```python
from build123d import *

# Parameters (mm, degrees)
F0_R     = 23.199373
F1_DEPTH = 12.7
F2_R     = 23.199373
F3_DEPTH = 12.7
F4_R     = 5.08


with BuildPart() as f1:
    # F0 (on Front) → F1 (new body)
    with BuildSketch(Plane.XZ):
        with Locations((-16.925193, -16.925193)):
            Circle(F0_R)
    extrude(amount=F1_DEPTH)

    # F2 (on face) → F3 (join)
    with BuildSketch(Plane(origin=(0, 0, 0), x_dir=(-1, 0, 0), z_dir=(0, 1, 0))):
        with Locations((16.925193, -16.925193)):
            Circle(F2_R)
    extrude(amount=F3_DEPTH)

    # F4
    f4_edges = [f1.edges().sort_by_distance(p)[0] for p in [
        (6.274179, 12.7, -16.925193),
        (-16.925193, 0, 6.274179),
        (-16.925193, 0, -40.124566),
        (6.274179, -6.35, -16.925193),
        (-40.124566, -12.7, -16.925193),
        (-40.124566, 6.35, -16.925193),
    ]]
    fillet(f4_edges, radius=F4_R)


solid = f1.part
```
Geometry: final body of the model. Coordinates: model frame, mm. Round coordinates to 2 decimals unless told otherwise and drop trailing zeros. Write each loop counter-clockwise with the first axis right and the second up, starting at its lowest first coordinate (ties: lowest second). Pieces come first, ordered by that corner, then holes. Notation, with made-up numbers: (-33.75, 49.5) -> (-13.75, 49.5) arc R24 ccw to (-13.75, 78.5) -> close; hole circle Ø9 at (81.25, 17). An arc over 180 degrees is marked (long way). Use CSV: the item, a comma, the result in double quotes. Start each with the question number.
Q1. Line query: L1, parallel to X at y = 10.5, z = -32; L2, parallel to Z at x = -28.5, y = 5.25; L3, parallel to Z at x = -14, y = 2. Output: solid intervals per line, ascending.
Q2. Section A-A (y = 10.25). Return loops of the section in (x, z), plus the area to 3 significant figures.
Q3. First-contact query: pin 1 Ø12 at (x, y) = (-20.5, 2) entering from -Z; pin 2 Ø8 at (y, z) = (-10, -8.5) entering from +X; pin 3 Ø8 at (x, y) = (-26.5, -4.5) entering from -Z. Flat tips, straight axial feed; report the tip coordinate or a pass-through.
Q4. Pull-direction query (Y, two-part tool) for faces 1 (the face through (-17, -12.7, -17)), 2 (the face through (-17, 12.7, -17)); classes: pulls with the +Y half, pulls with the -Y half, needs draft (parallel to the pull), parting line crosses it, or undercut.
Q5. Section B-B (y = 1.5). Return loops of the section in (x, z).
Result sheet:
1,L1,"-33.36 to -0.49"
1,L2,"-37.03 to 3.18"
1,L3,"-39.94 to 6.09"
2,outline,"circle Ø44.93 at (-16.93, -16.93)"
2,area,"1,590 mm²"
3,pin 1,"z = -40.12"
3,pin 2,"x = 5.73"
3,pin 3,"z = -39.44"
4,face 1,"pulls with the -Y half"
4,face 2,"pulls with the +Y half"
5,outline,"circle Ø46.4 at (-16.93, -16.93)"
